from build123d import *

# Parameters (mm, degrees)
SKETCH2_R           = 2.5
BOSS_EXTRUDE1_DEPTH = 25
SKETCH3_R           = 1
CUT_EXTRUDE1_DEPTH  = 25
SKETCH6_R           = 2.5
SKETCH6_W           = 20
SKETCH6_H           = 12.5
CUT_EXTRUDE2_DEPTH  = 144.01010212


with BuildPart() as part:
    # Sketch2 → Boss-Extrude1 (new body)
    with BuildSketch(Plane(origin=(0, 0, 0), x_dir=(1, 0, 0), z_dir=(0, 1, 0))):
        with BuildLine():
            Line((0.030237901, 33.847554993), (0.030237901, -135.452445007))
            ThreePointArc((0.030237901, -135.452445007), (7.071479353, -140.016799653), (8.363571234, -131.725665044))
            ThreePointArc((8.363571234, -131.725665044), (5.901528609, -128.354588024), (5.030237901, -124.272105119))
            Line((5.030237901, -124.272105119), (5.030237901, -71.632784894))
            ThreePointArc((5.030237901, -71.632784894), (5.901528609, -67.55030199), (8.363571234, -64.179224969))
            ThreePointArc((8.363571234, -64.179224969), (10.030237901, -60.452445007), (8.363571234, -56.725665044))
            ThreePointArc((8.363571234, -56.725665044), (5.901528609, -53.354588024), (5.030237901, -49.272105119))
            Line((5.030237901, -49.272105119), (5.030237901, -26.632784894))
            ThreePointArc((5.030237901, -26.632784894), (5.901528609, -22.55030199), (8.363571234, -19.179224969))
            ThreePointArc((8.363571234, -19.179224969), (10.030214165, -15.437038677), (8.340541648, -11.705194134))
            ThreePointArc((8.340541648, -11.705194134), (5.841334205, -8.313005826), (4.961165626, -4.192534659))
            Line((4.961165626, -4.192534659), (5.030237901, 33.847554993))
            Line((5.030237901, 33.847554993), (0.030237901, 33.847554993))
        make_face()
        with Locations(Location((5.030237901, -15.452445007, 0), (0, 0, 270))):
            Circle(SKETCH2_R, mode=Mode.SUBTRACT)
        with Locations(Location((5.030237901, -135.452445007, 0), (0, 0, 270))):
            Circle(SKETCH2_R, mode=Mode.SUBTRACT)
        with Locations(Location((5.030237901, -60.452445007, 0), (0, 0, 270))):
            Circle(SKETCH2_R, mode=Mode.SUBTRACT)
    extrude(amount=BOSS_EXTRUDE1_DEPTH)

    # Sketch3 → Cut-Extrude1 (cut)
    with BuildSketch(Plane(origin=(0, 0, -33.847554993), x_dir=(-1, 0, 0), z_dir=(0, 0, -1))):
        with Locations((-2.5, 15)):
            Circle(SKETCH3_R)
        with Locations((-2.5, 5)):
            Circle(SKETCH3_R)
    extrude(amount=-CUT_EXTRUDE1_DEPTH, mode=Mode.SUBTRACT)

    # Sketch6 → Cut-Extrude2 (cut, through all)
    with BuildSketch(Plane.ZY.offset(-0.030237901)):
        with Locations((40.98910992, 12.5)):
            Circle(SKETCH6_R)
        with Locations((60.98910992, 12.5)):
            Rectangle(SKETCH6_W, SKETCH6_H)
    extrude(amount=-CUT_EXTRUDE2_DEPTH, mode=Mode.SUBTRACT)


solid = part.part
Geometry: final body of the model. Coordinates: model frame, mm. A direction names the side the tool comes from. Round coordinates to 2 decimals unless told otherwise and drop trailing zeros. Order: outer loops, then holes, each group sorted by start corner. A loop starts at its lowest first (then second) coordinate and runs counter-clockwise, first axis right, second up.
Q1. Material intervals for probe 1 along Z at (x, y) = (2.75, 12); probe 2 along Z at (x, y) = (7.75, 22.25); probe 3 along Z at (x, y) = (3.75, 1), sorted ascending.
Result sheet:
probe 1: z = -33.85 to 14.43, 16.48 to 38.54, 43.44 to 50.99, 70.99 to 134.43, 136.48 to 139.9
probe 2: z = 11.14 to 19.78, 56.13 to 64.78, 131.13 to 139.65
probe 3: z = -33.85 to 13.31, 17.6 to 58.31, 62.6 to 133.31, 137.6 to 140.29
Q2. Section C-C, the plane z = 120. Output: boundary loops of the cut face in (x, y), and give its area (3 significant figures).
Result sheet:
outline: (0.03, 0) - (5.03, 0) - (5.03, 25) - (0.03, 25) - close
area: 125 mm2
Q3. Section B-B, the plane y = 22. Output: boundary loops of the cut face in (x, z).
Result sheet:
outline: (0.03, -33.85) - (5.03, -33.85) - (4.96, 4.19) arc R10 cw to (8.34, 11.71) arc R5 ccw to (8.36, 19.18) arc R10 cw to (5.03, 26.63) - (5.03, 49.27) arc R10 cw to (8.36, 56.73) arc R5 ccw to (8.36, 64.18) arc R10 cw to (5.03, 71.63) - (5.03, 124.27) arc R10 cw to (8.36, 131.73) arc R5 ccw (long way) to (0.03, 135.45) - close; hole circle Ø5 at (5.03, 15.45); hole circle Ø5 at (5.03, 60.45); hole circle Ø5 at (5.03, 135.45)
Q4. Pin query (flat end, axial travel): pin 1 (3 mm diameter, centred on x = 2.5, y = 15, fed in from +Z); pin 2 (7.5 mm diameter, centred on y = 9.5, z = 100.5, fed in from +X); pin 3 (2 mm diameter, centred on x = 2, y = 21, fed in from +Z). Return the tip coordinate at first contact, or that it passes through.
Result sheet:
pin 1: stops at z = 140.35
pin 2: stops at x = 5.03
pin 3: stops at z = 140.02
Q5. Mould query, pull axis Z, two halves, no side actions, for faces 4 (the face through (3, 12, -33.848)), 5 (the face through (3, 0, 52)), 6 (the face through (5.137, 12.325, 50.728)). Classes: released by +Z, released by -Z, zero draft, split by the parting line, or undercut.
Result sheet:
face 4: released by -Z
face 5: zero draft
face 6: undercut
Q6. Section D-D, the plane z = -13.5. Output: boundary loops of the cut face in (x, y), and give its area (3 significant figures).
Result sheet:
outline: (0.03, 0) - (4.99, 0) - (4.99, 25) - (0.03, 25) - close; hole circle Ø2 at (2.5, 5); hole circle Ø2 at (2.5, 15)
area: 118 mm2
Q7. Section A-A, the plane y = 12.5. Output: boundary loops of the cut face in (x, z), and give its area (3 significant figures).
Result sheet:
outline: (0.03, -33.85) - (5.03, -33.85) - (4.96, 4.19) arc R10 cw to (8.34, 11.71) arc R5 ccw to (8.36, 19.18) arc R10 cw to (5.03, 26.63) - (5.03, 38.49) - (0.03, 38.49) - close; (0.03, 43.49) - (5.03, 43.49) - (5.03, 49.27) arc R10 cw to (5.18, 50.99) - (0.03, 50.99) - close; (0.03, 70.99) - (5.05, 70.99) arc R10 cw to (5.03, 71.63) - (5.03, 124.27) arc R10 cw to (8.36, 131.73) arc R5 ccw (long way) to (0.03, 135.45) - close; hole circle Ø5 at (5.03, 15.45); hole circle Ø5 at (5.03, 135.45)
area: 793 mm2
Q8. Access query for faces 1 (the face through (3, 25, 52)), 2 (the face through (3, 12, 70.989)), 3 (the face through (5.03, 12, 98)). Directions: +Z, -Z, +X, -X, +Y, -Y. A direction counts if a zero-diameter tool reaches every point of the face in a straight line with its end or side. Return the directions, or none.
Result sheet:
face 1: +Z, -Z, +X, -X, +Y
face 2: +X, -X
face 3: +X, +Y, -Y
